```python
from build123d import *

# Parameters (mm, degrees)
SKETCH1_W           = 60
SKETCH1_H           = 93
BOSS_EXTRUDE1_DEPTH = 4
SKETCH3_R           = 1.65
CUT_EXTRUDE1_DEPTH  = 4
SKETCH5_W           = 60
SKETCH5_H           = 4
BOSS_EXTRUDE2_DEPTH = 11
SKETCH6_W           = 123.5
SKETCH6_H           = 4
BOSS_EXTRUDE3_DEPTH = 87.5
SKETCH7_R           = 1.65
CUT_EXTRUDE2_DEPTH  = 87.5
SKETCH10_R          = 1.65
CUT_EXTRUDE3_DEPTH  = 10
SKETCH11_W          = 98.5
SKETCH11_H          = 89
BOSS_EXTRUDE4_DEPTH = 25
SKETCH13_W          = 98.5
SKETCH13_H          = 89
CUT_EXTRUDE5_DEPTH  = 8
CUT_EXTRUDE7_DEPTH  = 20
SKETCH15_W          = 71.5
SKETCH15_H          = 17
BOSS_EXTRUDE6_DEPTH = 45
CUT_EXTRUDE9_DEPTH  = 45


with BuildPart() as part:
    # Sketch1 → Boss-Extrude1 (new body)
    with BuildSketch(Plane.XY):
        with Locations((30, -46.5)):
            Rectangle(SKETCH1_W, SKETCH1_H)
    extrude(amount=-BOSS_EXTRUDE1_DEPTH)

    # Sketch3 → Cut-Extrude1 (cut)
    with BuildSketch(Plane.XY):
        with Locations((4, -8)):
            Circle(SKETCH3_R)
        with Locations((56, -8)):
            Circle(SKETCH3_R)
        with Locations((4, -89)):
            Circle(SKETCH3_R)
        with Locations((56, -89)):
            Circle(SKETCH3_R)
    extrude(amount=-CUT_EXTRUDE1_DEPTH, mode=Mode.SUBTRACT)

    # Sketch5 → Boss-Extrude2 (add)
    with BuildSketch(Plane(origin=(0, 0, -4), x_dir=(-1, 0, 0), z_dir=(0, 0, -1))):
        with Locations((-30, -2)):
            Rectangle(SKETCH5_W, SKETCH5_H)
    extrude(amount=BOSS_EXTRUDE2_DEPTH)

    # Sketch6 → Boss-Extrude3 (add)
    with BuildSketch(Plane(origin=(0, 0, -15), x_dir=(-1, 0, 0), z_dir=(0, 0, -1))):
        with Locations((1.75, -2)):
            Rectangle(SKETCH6_W, SKETCH6_H)
    extrude(amount=BOSS_EXTRUDE3_DEPTH)

    # Sketch7 → Cut-Extrude2 (cut)
    with BuildSketch(Plane(origin=(0, 0, 0), x_dir=(1, 0, 0), z_dir=(0, 1, 0))):
        with Locations(Location((-59.5, 98.5, 0), (0, 0, 270))):
            Circle(SKETCH7_R)
        with Locations(Location((-36.5, 98.5, 0), (0, 0, 270))):
            Circle(SKETCH7_R)
        with Locations(Location((-59.5, 58.5, 0), (0, 0, 270))):
            Circle(SKETCH7_R)
        with Locations(Location((-36.5, 58.5, 0), (0, 0, 270))):
            Circle(SKETCH7_R)
    extrude(amount=-CUT_EXTRUDE2_DEPTH, mode=Mode.SUBTRACT)

    # Sketch10 → Cut-Extrude3 (cut)
    with BuildSketch(Plane(origin=(0, 0, 0), x_dir=(1, 0, 0), z_dir=(0, 1, 0))):
        with Locations(Location((29.5, 83.25, 0), (0, 0, 270))):
            Circle(SKETCH10_R)
        with Locations(Location((29.5, 56.75, 0), (0, 0, 270))):
            Circle(SKETCH10_R)
    extrude(amount=-CUT_EXTRUDE3_DEPTH, mode=Mode.SUBTRACT)

    # Sketch11 → Boss-Extrude4 (add)
    with BuildSketch(Plane(origin=(0, 0, 0), x_dir=(0, 0, -1), z_dir=(1, 0, 0))):
        with Locations((53.25, -48.5)):
            Rectangle(SKETCH11_W, SKETCH11_H)
    extrude(amount=BOSS_EXTRUDE4_DEPTH)

    # Sketch13 → Cut-Extrude5 (cut)
    with BuildSketch(Plane.ZY):
        with Locations((-53.25, -48.5)):
            Rectangle(SKETCH13_W, SKETCH13_H)
    extrude(amount=-CUT_EXTRUDE5_DEPTH, mode=Mode.SUBTRACT)

    # Sketch14 → Cut-Extrude7 (cut)
    with BuildSketch(Plane.ZY.offset(-8)):
        Polygon((-102.5, -4), (-102.5, -93), (-4, -93), align=None)
    extrude(amount=-CUT_EXTRUDE7_DEPTH, mode=Mode.SUBTRACT)

    # Sketch15 → Boss-Extrude6 (add)
    with BuildSketch(Plane.XZ.offset(4)):
        with Locations((-27.75, -42)):
            Rectangle(SKETCH15_W, SKETCH15_H)
    extrude(amount=BOSS_EXTRUDE6_DEPTH)

    # Sketch16 → Cut-Extrude9 (cut)
    with BuildSketch(Plane(origin=(0, 0, -50.5), x_dir=(-1, 0, 0), z_dir=(0, 0, -1))):
        Polygon((63.5, -4), (-8, -49), (63.5, -49), align=None)
    extrude(amount=-CUT_EXTRUDE9_DEPTH, mode=Mode.SUBTRACT)


solid = part.part
```
Work out the finished part from the listing and answer in its coordinate system (mm). A direction names the side the tool comes from. Round coordinates to 2 decimals unless told otherwise and drop trailing zeros. Write each loop counter-clockwise with the first axis right and the second up, starting at its lowest first coordinate (ties: lowest second). Pieces come first, ordered by that corner, then holes. Notation, with made-up numbers: (19.25, 88) -> (73.25, 88) arc R32 ccw to (73.25, 117) -> close; hole circle Ø6 at (86.5, 87). An arc over 180 degrees is marked (long way). Write each question's results on one line, items separated by ' | '.
Q1. Straight lines are drawn through the part: line 1 along Y through (x, z) = (56, -2); line 2 along X through (y, z) = (-89, -1); line 3 along X through (y, z) = (-1, -98). For each, find the intervals that lie inside material, in ascending order. Write a range as [from, to].
Data:
line 1: [-93, -90.65], [-87.35, -9.65], [-6.35, 0] | line 2: [0, 2.35], [5.65, 54.35], [57.65, 60] | line 3: [-63.5, -61.07], [-57.93, -38.07], [-34.93, 60]
Q2. Determine the mould class of faces 1 (the cylindrical face through (54.69, -90, -1.97)), 2 (the flat face through (30, -93, -2)), 3 (the flat face through (4, -49, -4)) for opening direction Y: released by +Y, released by -Y, zero draft, split by the parting line, or undercut.
Data:
face 1: undercut | face 2: released by -Y | face 3: zero draft
Q3. Section D-D, the plane z = -83.25 is taken. Write down the section's boundary in (x, y), then the cut area to 3 significant figures.
Data:
outline: (-63.5, -4) -> (8, -4) -> (8, -21.39) -> (25, -21.39) -> (25, -4) -> (27.85, -4) -> (27.85, 0) -> (-63.5, 0) -> close; (31.15, -4) -> (60, -4) -> (60, 0) -> (31.15, 0) -> close | area: 776 mm^2
Q4. Section A-A, the plane x = 56 is taken. Write down the section's boundary in (y, z).
Data:
outline: (-93, -4) -> (-90.65, -4) -> (-90.65, 0) -> (-93, 0) -> close; (-87.35, -4) -> (-9.65, -4) -> (-9.65, 0) -> (-87.35, 0) -> close; (-6.35, -4) -> (-4, -4) -> (-4, -102.5) -> (0, -102.5) -> (0, 0) -> (-6.35, 0) -> close
Q5. Flat-ended cylindrical pins translate along their axes: P1, Ø2, axis at x = 29.5, y = -46.5, coming from the +Z side; P2, Ø4, axis at x = 21.5, y = -45, coming from the -Z side; P3, Ø4, axis at x = -36.5, z = -58.5, coming from the -Y side; P4, Ø1, axis at y = -35, z = -64, coming from the -X side. Find the tip coordinate at first contact, or state that the pin passes through.
Data:
P1: z = 0 | P2: z = -59.34 | P3: y = -4 | P4: x = 8
Q6. Section B-B, the plane z = -98.5 is taken. Write down the section's boundary in (x, y), then the cut area to 3 significant figures.
Data:
outline: (-63.5, -4) -> (-61.15, -4) -> (-61.15, 0) -> (-63.5, 0) -> close; (-57.85, -4) -> (-38.15, -4) -> (-38.15, 0) -> (-57.85, 0) -> close; (-34.85, -4) -> (8, -4) -> (8, -7.61) -> (25, -7.61) -> (25, -4) -> (60, -4) -> (60, 0) -> (-34.85, 0) -> close | area: 529 mm^2
Q7. Section C-C, the plane y = -8 is taken. Write down the section's boundary in (x, z).
Data:
outline: (-57.14, -50.5) -> (8, -50.5) -> (8, -98.07) -> (25, -98.07) -> (25, -4) -> (54.35, -4) -> (54.35, 0) -> (5.65, 0) -> (5.65, -4) -> (8, -4) -> (8, -33.5) -> (-57.14, -33.5) -> close; (0, -4) -> (2.35, -4) -> (2.35, 0) -> (0, 0) -> close; (57.65, -4) -> (60, -4) -> (60, 0) -> (57.65, 0) -> close
Q8. Which of the six approach directions +Z, -Z, +X, -X, +Y, -Y give full straight-line access (tool end or side, diameter ignored) to faces 4 (the flat face through (43, -4, -53)), 5 (the flat face through (0, -43.3, -3.6)), 6 (the flat face through (-28, -4, -77)), 7 (the cylindrical face through (30.615, -1.972, -57.966)), 8 (the flat face through (-12, -16, -33.5))?
Data:
face 4: -Z, +X, -Y | face 5: +Z, -X, +Y, -Y | face 6: -Z, -X, -Y | face 7: +Y, -Y | face 8: -X, -Y
